The listing builds one solid part. Answer for the finished solid, in the listing's coordinates (mm). A direction names the side the tool comes from. Give positions to 0.01 mm unless a question says otherwise; leave off trailing zeros. Order: outer loops, then holes, each group sorted by start corner. A loop starts at its lowest first (then second) coordinate and runs counter-clockwise, first axis right, second up.
```python
from build123d import *

# Parameters (mm, degrees)
SKETCH1_W                    = 14.25702
SKETCH1_H                    = 25.4
SKETCH1_R                    = 3.175
BASE_FLANGE1_DEPTH           = 0.79375
EDGE_FLANGE1_DEPTH           = 25.4
EDGE_FLANGE2_DEPTH           = 25.4
EDGE_FLANGE3_DEPTH           = 25.4
EDGE_FLANGE4_STRIP_W         = 4.6482
EDGE_FLANGE4_STRIP_H         = 0.79375
EDGE_FLANGE4_STRIP_CUT_DEPTH = 25.4
EDGE_FLANGE4_DEPTH           = 25.4
SKETCH16_R                   = 3.175
CUT_EXTRUDE1_DEPTH           = 220.30417026
SKETCH19_W                   = 25.4
SKETCH19_H                   = 25.4
TAB1_DEPTH                   = 0.79375
EDGE_FLANGE5_STRIP_W         = 4.6482
EDGE_FLANGE5_STRIP_H         = 0.79375
EDGE_FLANGE5_STRIP_CUT_DEPTH = 25.4
EDGE_FLANGE5_DEPTH           = 25.4
SKETCH25_R                   = 3.96875
CUT_EXTRUDE2_DEPTH           = 228.075600106


# Sheet-metal steps are written as plain solids
with BuildPart() as part:
    # Sketch1 → Base-Flange1 (new body)
    with BuildSketch(Plane(origin=(0, 0, 0), x_dir=(1, 0, 0), z_dir=(0, 1, 0))):
        with Locations((-0.77851, 4.160748346)):
            Rectangle(SKETCH1_W, SKETCH1_H)
        with Locations(Location((0, 0, 0), (0, 0, 270))):
            Circle(SKETCH1_R, mode=Mode.SUBTRACT)
    extrude(amount=-BASE_FLANGE1_DEPTH)

    # Edge-Flange1 section (across the edge) → Edge-Flange1 (add)
    with BuildSketch(Plane(origin=(-8.64362, 0, -16.860748346), x_dir=(1, 0, 0), z_dir=(0, 0, 1))):
        with BuildLine():
            Line((-0.79375, 0.7366), (-0.79375, 9.9949))
            Line((-0.79375, 9.9949), (0, 9.9949))
            Line((0, 9.9949), (0, 0.7366))
            ThreePointArc((0, 0.7366), (0.215745145, 0.215745145), (0.7366, 0))
            Line((0.7366, 0), (0.7366, -0.79375))
            ThreePointArc((0.7366, -0.79375), (-0.345520863, -0.345520863), (-0.79375, 0.7366))
        make_face()
    extrude(amount=EDGE_FLANGE1_DEPTH)

    # Edge-Flange2 section (across the edge) → Edge-Flange2 (add)
    with BuildSketch(Plane(origin=(-9.43737, 10.7315, 8.539251654), x_dir=(0, -1, 0), z_dir=(0, 0, -1))):
        with BuildLine():
            Line((-0.79375, 0.7366), (-0.79375, 192.38595))
            Line((-0.79375, 192.38595), (0, 192.38595))
            Line((0, 192.38595), (0, 0.7366))
            ThreePointArc((0, 0.7366), (0.215745145, 0.215745145), (0.7366, 0))
            Line((0.7366, 0), (0.7366, -0.79375))
            ThreePointArc((0.7366, -0.79375), (-0.345520863, -0.345520863), (-0.79375, 0.7366))
        make_face()
    extrude(amount=EDGE_FLANGE2_DEPTH)

    # Edge-Flange3 section (across the edge) → Edge-Flange3 (add)
    with BuildSketch(Plane(origin=(-202.55992, 10.7315, 8.539251654), x_dir=(1, 0, 0), z_dir=(0, 0, -1))):
        with BuildLine():
            Line((-0.79375, 0.7366), (-0.79375, 11.52525))
            Line((-0.79375, 11.52525), (0, 11.52525))
            Line((0, 11.52525), (0, 0.7366))
            ThreePointArc((0, 0.7366), (0.215745145, 0.215745145), (0.7366, 0))
            Line((0.7366, 0), (0.7366, -0.79375))
            ThreePointArc((0.7366, -0.79375), (-0.345520863, -0.345520863), (-0.79375, 0.7366))
        make_face()
    extrude(amount=EDGE_FLANGE3_DEPTH)

    # Edge-Flange4 strip (across the edge) → Edge-Flange4 strip cut (cut)
    with BuildSketch(Plane(origin=(-203.35367, -0.79375, -16.860748346), x_dir=(0, 1, 0), z_dir=(0, 0, 1))):
        with Locations((-0.79375, -0.396875)):
            Rectangle(EDGE_FLANGE4_STRIP_W, EDGE_FLANGE4_STRIP_H)
    extrude(amount=EDGE_FLANGE4_STRIP_CUT_DEPTH, mode=Mode.SUBTRACT)

    # Edge-Flange4 section (across the edge) → Edge-Flange4 (add)
    with BuildSketch(Plane(origin=(-203.35367, -0.79375, -16.860748346), x_dir=(0, 1, 0), z_dir=(0, 0, 1))):
        with BuildLine():
            Line((0, 0.7366), (0, 14.99743))
            Line((0, 14.99743), (0.79375, 14.99743))
            Line((0.79375, 14.99743), (0.79375, 0.7366))
            ThreePointArc((0.79375, 0.7366), (1.009495145, 0.215745145), (1.53035, 0))
            Line((1.53035, 0), (1.53035, -0.79375))
            ThreePointArc((1.53035, -0.79375), (0.448229137, -0.345520863), (0, 0.7366))
        make_face()
    extrude(amount=EDGE_FLANGE4_DEPTH)

    # Sketch16 → Cut-Extrude1 (cut, through all)
    with BuildSketch(Plane(origin=(0, 0, 0), x_dir=(1, 0, 0), z_dir=(0, 1, 0))):
        with Locations(Location((-211.998031426, 0, 0), (0, 0, 180))):
            Circle(SKETCH16_R)
    extrude(amount=-CUT_EXTRUDE1_DEPTH, mode=Mode.SUBTRACT)

    # Sketch19 → Tab1 (add)
    with BuildSketch(Plane(origin=(0, 11.52525, 0), x_dir=(1, 0, 0), z_dir=(0, 1, 0))):
        with Locations((-31.75, -21.239251654)):
            Rectangle(SKETCH19_W, SKETCH19_H)
    extrude(amount=-TAB1_DEPTH)

    # Edge-Flange5 strip (across the edge) → Edge-Flange5 strip cut (cut)
    with BuildSketch(Plane(origin=(-44.45, 11.52525, 33.939251654), x_dir=(0, 0, -1), z_dir=(1, 0, 0))):
        with Locations((-0.79375, -0.396875)):
            Rectangle(EDGE_FLANGE5_STRIP_W, EDGE_FLANGE5_STRIP_H)
    extrude(amount=EDGE_FLANGE5_STRIP_CUT_DEPTH, mode=Mode.SUBTRACT)

    # Edge-Flange5 section (across the edge) → Edge-Flange5 (add)
    with BuildSketch(Plane(origin=(-44.45, 11.52525, 33.939251654), x_dir=(0, 0, -1), z_dir=(1, 0, 0))):
        with BuildLine():
            Line((0, 0.7366), (0, 24.60625))
            Line((0, 24.60625), (0.79375, 24.60625))
            Line((0.79375, 24.60625), (0.79375, 0.7366))
            ThreePointArc((0.79375, 0.7366), (1.009495145, 0.215745145), (1.53035, 0))
            Line((1.53035, 0), (1.53035, -0.79375))
            ThreePointArc((1.53035, -0.79375), (0.448229137, -0.345520863), (0, 0.7366))
        make_face()
    extrude(amount=EDGE_FLANGE5_DEPTH)

    # Sketch25 → Cut-Extrude2 (cut, through all)
    with BuildSketch(Plane.XY.offset(33.939251654)):
        with Locations((-31.75, 24.96185)):
            Circle(SKETCH25_R)
    extrude(amount=-CUT_EXTRUDE2_DEPTH, mode=Mode.SUBTRACT)


solid = part.part
```
1) Find section D-D (x = 0). Write down the section's boundary in (y, z) (3 decimals).
Geometry says:
outline: (-0.794, -16.861) - (0, -16.861) - (0, -3.175) - (-0.794, -3.175) - close; (-0.794, 3.175) - (0, 3.175) - (0, 8.539) - (-0.794, 8.539) - close
2) Straight lines are drawn through the part: probe 1 along Y at (x, z) = (-38, -14); probe 2 along X at (y, z) = (11, 21.5). For each, find the intervals that lie inside material, in ascending order.
Geometry says:
probe 1: y = 10.73 to 11.53
probe 2: x = -44.45 to -19.05
3) Find section B-B (x = -31.75). Write down the section's boundary in (y, z), then the cut area to 3 significant figures.
Geometry says:
outline: (10.73, -16.86) - (11.53, -16.86) - (11.53, 32.41) arc R0.74 cw to (12.26, 33.15) - (20.99, 33.15) - (20.99, 33.94) - (12.26, 33.94) arc R1.53 ccw to (10.73, 32.41) - close; (28.93, 33.15) - (36.13, 33.15) - (36.13, 33.94) - (28.93, 33.94) - close
area: 53.2 mm2
4) Given P1, Ø7.5, axis at x = -212, z = 0, coming from the +Y side; P2, Ø6, axis at x = -174, z = 0.5, coming from the -Y side; P3, Ø4.5, axis at y = 5, z = -4, coming from the -X side, each flat-ended and moving along its own axis, determine where each tip first touches the part or whether it passes through.
Geometry says:
P1: stops at y = 0
P2: stops at y = 10.73
P3: stops at x = -203.35
5) Find section A-A (y = 7.5). Write down the section's boundary in (x, z), then the cut area to 3 significant figures.
Geometry says:
outline: (-203.35, -16.86) - (-202.56, -16.86) - (-202.56, 8.54) - (-203.35, 8.54) - close; (-9.44, -16.86) - (-8.64, -16.86) - (-8.64, 8.54) - (-9.44, 8.54) - close
area: 40.3 mm2
6) A tool of negligible diameter and unlimited length cuts with its end or side. For faces 1 (the flat face through (-202.56, 5, -4)), 2 (the flat face through (-83, 11.525, 3)), 3 (the flat face through (-44.45, 11, 27)), 4 (the flat face through (-9, 4, 8.539)), from which of +Z, -Z, +X, -X, +Y, -Y can it reach the whole face along a straight path? Write none if from no direction.
Geometry says:
face 1: +Z, -Z, -Y
face 2: -Z, +X, -X, +Y
face 3: +Z, -X, +Y, -Y
face 4: +Z, +X, +Y, -Y
7) For a pull along X with two mould halves and no side action, classify faces 5 (the flat face through (-19.05, 11, 27)), 6 (the cylindrical face through (-209.66, -0.39, 2.15)), 7 (the flat face through (-203.354, 5, -4)), 8 (the flat face through (-211, -0.794, -4)) as +X half, -X half, draft (parallel to the pull), parting line (faces both ways), or undercut.
Geometry says:
face 5: +X half
face 6: undercut
face 7: -X half
face 8: draft
8) Find section C-C (z = 0). Count the separate pieces of the cut face and the enclosed holes in it, then the cut area to 3 significant figures.
Geometry says:
separate pieces: 3
enclosed holes: 0
area: 185 mm2
